from build123d import *

# Parameters (mm, degrees)
F0_R     = 11.1155463884
F1_DEPTH = 19.05
F2_R     = 1.27


with BuildPart() as f1:
    # F0 (on Front) → F1 (new body)
    with BuildSketch(Plane.XZ):
        with BuildLine():
            add(Edge.make_bspline(
                [(-38.1638994336, 0), (-19.6957219024, 2.1979471251), (-9.311880126, 4.0390839853), (-2.7506002225, 14.761891216), (0, 19.05)],
                knots=[0, 0, 0, 0, 0.5912055263, 1, 1, 1, 1], degree=3))
            add(Edge.make_bspline(
                [(-13.9198412699, -11.1125), (-14.794313883, -9.2288451722), (-17.1100002201, -4.2407487086), (-39.5685055328, -1.9231498725), (-38.3696140076, -0.2816590053), (-38.1638994336, 0)],
                knots=[0, 0, 0, 0, 0.3345084593, 0.8858100955, 1, 1, 1, 1], degree=3))
            ThreePointArc((-13.9198412699, -11.1125), (0, -20.7508764), (13.9198412699, -11.1125))
            add(Edge.make_bspline(
                [(13.9198412699, -11.1125), (14.8240544816, -9.1946143672), (17.2053802942, -4.1436921907), (39.2933100068, -2.4877446669), (38.244207933, -0.4117993191), (38.0361005664, 0)],
                knots=[0, 0, 0, 0, 0.3291827069, 0.8669318993, 1, 1, 1, 1], degree=3))
            add(Edge.make_bspline(
                [(38.0361005664, 0), (20.2584086937, 2.241044324), (10.7040125651, 3.3870131368), (2.4307208404, 14.9494804331), (0, 19.05)],
                knots=[0, 0, 0, 0, 0.5801098598, 1, 1, 1, 1], degree=3))
        make_face()
        with Locations((0, -6.0836733319)):
            Circle(F0_R, mode=Mode.SUBTRACT)
    extrude(amount=F1_DEPTH)

    # F2
    f2_edges = [f1.edges().sort_by_distance(p)[0] for p in [
        (15.828231, -19.05, 3.702963),
        (15.828231, 0, 3.702963),
        (-15.834222, -19.05, 3.677027),
        (-15.834222, 0, 3.677027),
    ]]
    fillet(f2_edges, radius=F2_R)


solid = f1.part
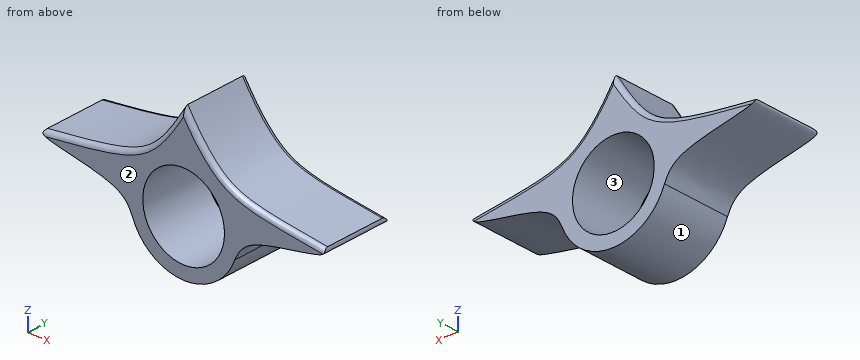
Work out the finished part from the listing and answer in its coordinate system (mm). Face numbers are marked on the shaded views. Coordinates: 2 decimals unless noted, no trailing zeros. Loops run counter-clockwise (first coordinate to the right, second up) from the corner with the lowest first, then second, coordinate; pieces in that order, holes last. Notation, with made-up numbers: (32.25, 11) -> (47.25, 11) arc R24 ccw to (47.25, 38) -> close; hole circle Ø2 at (53.25, 25). An arc over 180 degrees is marked (long way). Write each question's results on one line, items separated by ' | '. Start each with the question number.
1) The mould has two halves that part along X. Classify the marked faces 1, 2 and 3: pulls with the +X half, pulls with the -X half, needs draft (parallel to the pull), parting line crosses it, or undercut.
2) Consider line 1 along Z through (x, y) = (-4, -6.5); line 2 along X through (y, z) = (-15, -9); line 3 along Y through (x, z) = (-0.5, 16). Determine where each line is inside the solid, lowest interval first.
3) Find section A-A on z = -15.5. Determine the outline of the cut face in (x, y), then the cut area to 3 significant figures.
4) Flat-ended cylindrical pins translate along their axes: P1, Ø1.5, axis at y = -6, z = -13.5, coming from the -X side; P2, Ø6, axis at x = -24, y = -11, coming from the -Z side; P3, Ø1, axis at x = 8, z = 1.5, coming from the +Y side; P4, Ø2, axis at x = 18.5, y = -2, coming from the +Z side. Find the tip coordinate at first contact, or state that the pin passes through.
Response values:
1) face 1: parting line crosses it | face 2: needs draft | face 3: undercut
2) line 1: z = -20.2 to -16.45, 4.29 to 12.97 | line 2: x = -15.05 to -10.73, 10.73 to 15.05 | line 3: y = -19.05 to 0
3) outline: (-11.34, -19.05) -> (-5.91, -19.05) -> (-5.91, 0) -> (-11.34, 0) -> close; (5.91, -19.05) -> (11.34, -19.05) -> (11.34, 0) -> (5.91, 0) -> close | area: 207 mm^2
4) P1: stops at x = -13.19 | P2: stops at z = -5.16 | P3: stops at y = 0 | P4: stops at z = 3.2
